Build history of the part. All positions in model axes, mm. A direction names the side the tool comes from. Round coordinates to 2 decimals unless told otherwise and drop trailing zeros. Order: outer loops, then holes, each group sorted by start corner. A loop starts at its lowest first (then second) coordinate and runs counter-clockwise, first axis right, second up. Notation, with made-up numbers: (64, -15.5) -> (74, -15.5) arc R18 ccw to (74, 13.5) -> close; hole circle Ø7 at (39, -1). An arc over 180 degrees is marked (long way). Write item = value, one per line.
from build123d import *

# Parameters (mm, degrees)
SKICA1_W                 = 62.391596743
SKICA1_H                 = 24
P_IDAT_VYSUNUT_M1_DEPTH  = 4
SKICA2_W                 = 42.3
SKICA2_H                 = 5
P_IDAT_VYSUNUT_M2_DEPTH  = 16
SKICA3_R                 = 1.6
SKICA3_R_2               = 12.36434098
P_IDAT_VYSUNUT_M5_DEPTH  = 5
ZKOSEN_1_SIZE            = 16
SKICA4_R                 = 2.6
ODEBRAT_VYSUNUT_M1_DEPTH = 4
SKICA5_W                 = 62.391596743
SKICA5_H                 = 4
P_IDAT_VYSUNUT_M6_DEPTH  = 20
SKICA6_R                 = 2.6
ODEBRAT_VYSUNUT_M2_DEPTH = 4


with BuildPart() as part:
    # Skica1 → Přidat vysunutím1 (new body)
    with BuildSketch(Plane.XY):
        with Locations((-71.195798372, -0.971059771)):
            Rectangle(SKICA1_W, SKICA1_H)
    extrude(amount=P_IDAT_VYSUNUT_M1_DEPTH)

    # Skica2 → Přidat vysunutím2 (add)
    with BuildSketch(Plane.XY.offset(4)):
        with Locations((-61.15, 8.528940229)):
            Rectangle(SKICA2_W, SKICA2_H)
    extrude(amount=P_IDAT_VYSUNUT_M2_DEPTH)

    # Skica3 → Přidat vysunutím5 (add)
    with BuildSketch(Plane.XY.offset(20)):
        Polygon((-40, 6.028940229), (-82.3, 6.028940229), (-82.3, 49.328940229), (-78.3, 53.328940229), (-44, 53.328940229), (-40, 49.328940229), align=None)
        with Locations((-45.65, 47.678940229)):
            Circle(SKICA3_R, mode=Mode.SUBTRACT)
        with Locations((-76.65, 47.678940229)):
            Circle(SKICA3_R, mode=Mode.SUBTRACT)
        with Locations((-76.65, 16.678940229)):
            Circle(SKICA3_R, mode=Mode.SUBTRACT)
        with Locations((-45.65, 16.678940229)):
            Circle(SKICA3_R, mode=Mode.SUBTRACT)
        with Locations((-61.15, 32.178940229)):
            Circle(SKICA3_R_2, mode=Mode.SUBTRACT)
    extrude(amount=P_IDAT_VYSUNUT_M5_DEPTH)

    # Zkosení1
    zkosen_1_edges = [part.edges().sort_by_distance(p)[0] for p in [
        (-82.3, 8.528940229, 4),
    ]]
    chamfer(zkosen_1_edges, length=ZKOSEN_1_SIZE)

    # Skica4 → Odebrat vysunutím1 (cut)
    with BuildSketch(Plane.XY.offset(4)):
        with Locations((-89.655606689, -2.971059771)):
            Circle(SKICA4_R)
        with Locations((-69.655606689, -2.971059771)):
            Circle(SKICA4_R)
        with Locations((-49.655606689, -2.971059771)):
            Circle(SKICA4_R)
    extrude(amount=-ODEBRAT_VYSUNUT_M1_DEPTH, mode=Mode.SUBTRACT)

    # Skica5 → Přidat vysunutím6 (add)
    with BuildSketch(Plane(origin=(0, 0, 0), x_dir=(-1, 0, 0), z_dir=(0, 0, -1))):
        with Locations((71.195798372, 9.028940229)):
            Rectangle(SKICA5_W, SKICA5_H)
    extrude(amount=P_IDAT_VYSUNUT_M6_DEPTH)

    # Skica6 → Odebrat vysunutím2 (cut)
    with BuildSketch(Plane(origin=(0, 11.028940229, 0), x_dir=(1, 0, 0), z_dir=(0, 1, 0))):
        with Locations(Location((-92.391596743, 10, 0), (0, 0, 270))):
            Circle(SKICA6_R)
    extrude(amount=-ODEBRAT_VYSUNUT_M2_DEPTH, mode=Mode.SUBTRACT)


solid = part.part
Q1. Which spindle directions (+Z, -Z, +X, -X, +Y, -Y) get a long thin tool onto all of the face, cutting with end or side? Do faces 1 (the face through (-62, 6.029, 14)), 2 (the face through (-80.33, 51.3, 22.46)), 3 (the face through (-72, -1, 0)). Say none if no direction does.
Check values:
face_1 = +Z, +X, -X, -Y
face_2 = +Z, -Z, -X, +Y
face_3 = -Z, +X, -X, -Y
Q2. Cut at A-A, the plane x = -76.65. List the corners of the cut face in (y, z).
Check values:
outline = (-12.97, 0) -> (7.03, 0) -> (7.03, -20) -> (11.03, -20) -> (11.03, 20) -> (15.08, 20) -> (15.08, 25) -> (6.03, 25) -> (6.03, 4) -> (-12.97, 4) -> close; (18.28, 20) -> (46.08, 20) -> (46.08, 25) -> (18.28, 25) -> close; (49.28, 20) -> (53.33, 20) -> (53.33, 25) -> (49.28, 25) -> close
Q3. Cut at D-D, the plane y = 21. List the corners of the cut face in (x, z).
Check values:
outline = (-82.3, 20) -> (-66.43, 20) -> (-66.43, 25) -> (-82.3, 25) -> close; (-55.87, 20) -> (-40, 20) -> (-40, 25) -> (-55.87, 25) -> close
Q4. Cut at B-B, the plane z = -10. List the corners of the cut face in (x, y).
Check values:
outline = (-102.39, 7.03) -> (-94.99, 7.03) -> (-94.99, 11.03) -> (-102.39, 11.03) -> close; (-89.79, 7.03) -> (-40, 7.03) -> (-40, 11.03) -> (-89.79, 11.03) -> close
Q5. Flat gauge pins, fed straight in: pin 1 (7 mm diameter, centred on x = -89.66, y = -2.97, fed in from -Z); pin 2 (5 mm diameter, centred on x = -45.65, y = 47.68, fed in from -Z); pin 3 (2.5 mm diameter, centred on y = 36, z = 21.5, fed in from -X); pin 4 (4.5 mm diameter, centred on x = -49.66, y = -2.97, fed in from -Z). Where does each tip first touch, or does it go through?
Check values:
pin_1 = 0
pin_2 = 20
pin_3 = -82.3
pin_4 = through
Q6. Mould opens along X. For faces 4 (the face through (-40, 9, 13)), 5 (the face through (-47.176, -2.19, 2.028)), 6 (the face through (-75.124, 48.16, 22.465)), 7 (the face through (-71, 11.029, 0)) say: released by +X, released by -X, zero draft, split by the parting line, or undercut.
Check values:
face_4 = released by +X
face_5 = undercut
face_6 = undercut
face_7 = zero draft
Q7. Cut at C-C, the plane x = -61.15. List the corners of the cut face in (y, z).
Check values:
outline = (-12.97, 0) -> (7.03, 0) -> (7.03, -20) -> (11.03, -20) -> (11.03, 20) -> (19.81, 20) -> (19.81, 25) -> (6.03, 25) -> (6.03, 4) -> (-12.97, 4) -> close; (44.54, 20) -> (53.33, 20) -> (53.33, 25) -> (44.54, 25) -> close
Q8. Probe probe 1 along Y at (x, z) = (-45.65, 23.15); probe 2 along Y at (x, z) = (-76, 21); probe 3 along Y at (x, z) = (-61, 23). List the from-to ranges inside material, lowest first.
Check values:
probe_1 = 6.03 to 15.08, 18.28 to 46.08, 49.28 to 53.33
probe_2 = 6.03 to 15.22, 18.14 to 46.22, 49.14 to 53.33
probe_3 = 6.03 to 19.82, 44.54 to 53.33
